Autodesk Inventor part; units mm, degrees
ref_plane "YZ Plane" through (0, 0, 0) normal (1, 0, 0) x (0, 1, 0)
ref_plane "XZ Plane" through (0, 0, 0) normal (0, 1, 0) x (-1, 0, 0)
ref_plane "XY Plane" through (0, 0, 0) normal (0, 0, 1) x (1, 0, 0)
sketch "Эскиз1" plane through (0, 0, 0) normal (0, 0, 1) x (1, 0, 0)
  arc A0 (-5.5627, -2.2486) -> (5.5627, 2.2486) centre (0, 0) ccw
  circle A1 centre (-114.2699, 282.6835) radius 2.5
  arc A2 (-108.7072, 284.9321) -> (-119.8326, 280.4348) centre (-114.2699, 282.6835) ccw
  arc A3 (-107.4093, 285.4568) -> (-121.1306, 279.9102) centre (-114.2699, 282.6835) ccw
  line L0 (-107.4093, 285.4568) -> (6.8607, 2.7733)
  line L1 (-6.8607, -2.7733) -> (-121.1306, 279.9102)
  line L2 (5.5627, 2.2486) -> (-108.7072, 284.9321)
  line L3 (-119.8326, 280.4348) -> (-5.5627, -2.2486)
  arc A4 (-6.8607, -2.7733) -> (6.8607, 2.7733) centre (0, 0) ccw
  dimension "d0" = 12
  dimension "d1" = 1.4
  dimension "d3" = 12
  dimension "d4" = 1.4
extrude "Выдавливание1" add sketch "Эскиз1" along normal mid plane 6 contours L0 A4 L1 A3
properties part number "ремень оси y"
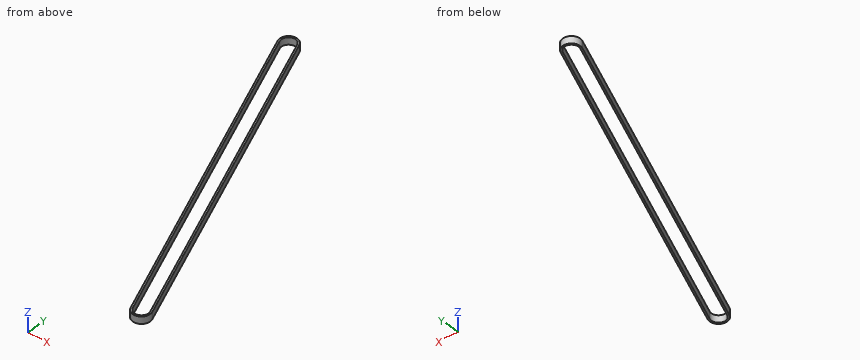
Source: CAD feature listing. Evaluate the final solid. Frame: model axes, mm. Give positions to 0.01 mm unless a question says otherwise; leave off trailing zeros. Loops run counter-clockwise (first coordinate to the right, second up) from the corner with the lowest first, then second, coordinate; pieces in that order, holes last. Notation, with made-up numbers: (49.25, 54) - (59.25, 54) arc R21 cw to (59.25, 91) - close; hole circle Ø2 at (47.25, -17.75). An arc over 180 degrees is marked (long way). Use CSV: the item, a comma, the result in double quotes.
1) Cut plane A-A (z = -1.8). Output: boundary loops of the cut face in (x, y), and give its area (3 significant figures).
Worked out:
outline,"(-121.13, 279.91) - (-6.86, -2.77) arc R7.4 ccw to (6.86, 2.77) - (-107.41, 285.46) arc R7.4 ccw to start; hole (-119.83, 280.43) - (-5.56, -2.25) arc R6 ccw to (5.56, 2.25) - (-108.71, 284.93) arc R6 ccw to start"
area,"913 mm^2"
2) Line query: line 1 (Y direction, x = -44, z = -1.35); line 2 (Y direction, x = -86, z = 0.05); line 3 (X direction, y = 215.5, z = -2). Output: solid intervals per line, ascending.
Worked out:
line 1,"y = 89.1 to 92.84, 124.86 to 128.59"
line 2,"y = 193 to 196.74, 228.76 to 232.49"
line 3,"x = -95.09 to -93.58, -80.64 to -79.13"
3) Pin query (flat end, axial travel): P1, Ø1.5, axis at x = -59, z = -2, coming from the +Y side. Return the tip coordinate at first contact, or that it passes through.
Worked out:
P1,"stops at y = 167.56"
4) Cut plane C-C (x = -27). Output: boundary loops of the cut face in (y, z), and give its area (3 significant figures).
Worked out:
outline,"(47.05, -3) - (50.78, -3) - (50.78, 3) - (47.05, 3) - close; (82.8, -3) - (86.54, -3) - (86.54, 3) - (82.8, 3) - close"
area,"44.8 mm^2"
5) Cut plane B-B (y = 23.5). Output: boundary loops of the cut face in (x, z).
Worked out:
outline,"(-17.48, -3) - (-15.97, -3) - (-15.97, 3) - (-17.48, 3) - close; (-3.03, -3) - (-1.52, -3) - (-1.52, 3) - (-3.03, 3) - close"
